Geometry check sheet. Reference: the model listing, model coordinates, mm. Round coordinates to 2 decimals unless told otherwise and drop trailing zeros. Write each loop counter-clockwise with the first axis right and the second up, starting at its lowest first coordinate (ties: lowest second). Pieces come first, ordered by that corner, then holes. Notation, with made-up numbers: (70.5, 16.5) - (98.5, 16.5) arc R13 cw to (98.5, 28.5) - close; hole circle Ø3 at (-22.5, 31). An arc over 180 degrees is marked (long way). Return JSON: item names as keys, results as strings.
```python
from build123d import *

# Parameters (mm, degrees)
SKETCH014_W            = 103
SKETCH014_H            = 207
PAD006_DEPTH           = 18
POCKET008_DEPTH        = 16
LINEARPATTERN_COUNT    = 4
LINEARPATTERN_PITCH    = 18
POCKET009_DEPTH        = 16
LINEARPATTERN001_COUNT = 2
LINEARPATTERN001_PITCH = 24
POCKET010_DEPTH        = 11.5
SKETCH019_W            = 55
SKETCH019_H            = 79
POCKET011_DEPTH        = 15
POCKET012_DEPTH        = 100
POCKET012_DEPTH_BACK   = 100
POCKET013_DEPTH        = 16
FILLET003_R            = 1
FILLET004_R            = 5
FILLET005_R            = 1
FILLET006_R            = 0.75


with BuildPart() as part:
    # Sketch014 → Pad006 (new body)
    with BuildSketch(Plane.XY):
        Rectangle(SKETCH014_W, SKETCH014_H)
    extrude(amount=PAD006_DEPTH)

    # Sketch015 (on Face6 of Pad006) → Pocket008 (cut)
    with BuildSketch(Plane(origin=(0, 90, 18), x_dir=(1, 0, 0), z_dir=(0, 0, 1))):
        with BuildLine():
            ThreePointArc((-40, 8), (-48, 0), (-40, -8))
            Line((-40, -8), (40, -8))
            ThreePointArc((40, -8), (48, 0), (40, 8))
            Line((-40, 8), (40, 8))
        make_face()
    pocket008 = extrude(amount=-POCKET008_DEPTH, mode=Mode.SUBTRACT)

    # LinearPattern: Pocket008 ×4
    with Locations(*[(0, -i * LINEARPATTERN_PITCH, 0) for i in range(1, LINEARPATTERN_COUNT)]):
        add(pocket008, mode=Mode.SUBTRACT)

    # Sketch017 → Pocket009 (cut)
    with BuildSketch(Plane(origin=(-15, 15, 18), x_dir=(1, 0, 0), z_dir=(0, 0, 1))):
        with BuildLine():
            Line((-23.5, 11), (23.5, 11))
            Line((23.5, 11), (15.797717, 0))
            Line((15.797717, 0), (23.5, -11))
            Line((23.5, -11), (-23.5, -11))
            ThreePointArc((-23.5, 11), (-34.5, 0), (-23.5, -11))
        make_face()
    pocket009 = extrude(amount=-POCKET009_DEPTH, mode=Mode.SUBTRACT)

    # LinearPattern001: Pocket009 ×2
    with Locations(*[(0, -i * LINEARPATTERN001_PITCH, 0) for i in range(1, LINEARPATTERN001_COUNT)]):
        add(pocket009, mode=Mode.SUBTRACT)

    # Sketch018 (on Face5 of LinearPattern001) → Pocket010 (cut)
    with BuildSketch(Plane.XY.offset(18)):
        with BuildLine():
            Line((48.255785, 16.86923), (48.255785, -41.13077))
            Line((48.255785, -41.13077), (43.255785, -41.13077))
            ThreePointArc((24.255785, -41.13077), (33.755784, -50.63077), (43.255785, -41.13077))
            Line((24.255785, -41.13077), (19.255785, -41.13077))
            Line((19.255785, -41.13077), (19.255785, 16.86923))
            Line((24.255785, 16.86923), (19.255785, 16.86923))
            ThreePointArc((43.255785, 16.86923), (33.755785, 26.36923), (24.255785, 16.86923))
            Line((43.255785, 16.86923), (48.255785, 16.86923))
        make_face()
    extrude(amount=-POCKET010_DEPTH, mode=Mode.SUBTRACT)

    # Sketch019 (on Face5 of Pocket010) → Pocket011 (cut)
    with BuildSketch(Plane.XY.offset(18)):
        with Locations((-22, -62)):
            Rectangle(SKETCH019_W, SKETCH019_H)
    extrude(amount=-POCKET011_DEPTH, mode=Mode.SUBTRACT)

    # Sketch020 (on Face46 of Pocket011) → Pocket012 (cut, two sides)
    with BuildSketch(Plane.XY.offset(3)) as pocket012_sk:
        with BuildLine():
            ThreePointArc((-35.75, -103.5), (-22, -117.25), (-8.25, -103.5))
            Line((-8.25, -103.5), (-8.25, -77.166667))
            ThreePointArc((-8.25, -77.166667), (-22, -63.416667), (-35.75, -77.166667))
            Line((-35.75, -103.5), (-35.75, -77.166667))
        make_face()
    extrude(amount=-POCKET012_DEPTH, mode=Mode.SUBTRACT)
    extrude(pocket012_sk.sketch, amount=POCKET012_DEPTH_BACK, mode=Mode.SUBTRACT)

    # Sketch021 (on Face5 of Pocket012) → Pocket013 (cut)
    with BuildSketch(Plane.XY.offset(18)):
        with BuildLine():
            ThreePointArc((7.5, -80.504131), (28.5, -101.504131), (49.5, -80.504131))
            Line((49.5, -80.504131), (49.5, -73.202981))
            ThreePointArc((49.5, -73.202981), (28.5, -52.202981), (7.5, -73.202981))
            Line((7.5, -80.504131), (7.5, -73.202981))
        make_face()
    extrude(amount=-POCKET013_DEPTH, mode=Mode.SUBTRACT)

    # Fillet003
    fillet003_edges = [part.edges().sort_by_distance(p)[0] for p in [
        (-42.625, -101.5, 18),
        (-49.5, -62, 18),
        (-22, -22.5, 18),
        (5.5, -62, 18),
        (-1.375, -101.5, 18),
    ]]
    fillet(fillet003_edges, radius=FILLET003_R)

    # Fillet004
    fillet004_edges = [part.edges().sort_by_distance(p)[0] for p in [
        (28.5, -52.202981, 2),
    ]]
    fillet(fillet004_edges, radius=FILLET004_R)

    # Fillet005
    fillet005_edges = [part.edges().sort_by_distance(p)[0] for p in [
        (48.255785, -12.13077, 18),
        (19.255785, -12.13077, 18),
    ]]
    fillet(fillet005_edges, radius=FILLET005_R)

    # Fillet006
    fillet006_edges = [part.edges().sort_by_distance(p)[0] for p in [
        (0, 80, 18),
        (-48, 72, 18),
        (0, 64, 18),
        (48, 72, 18),
        (0, 62, 18),
        (-48, 54, 18),
        (0, 46, 18),
        (48, 54, 18),
        (0, 44, 18),
        (-48, 36, 18),
        (0, 28, 18),
        (48, 36, 18),
        (0, 98, 18),
        (-48, 90, 18),
        (0, 82, 18),
        (48, 90, 18),
    ]]
    fillet(fillet006_edges, radius=FILLET006_R)


solid = part.part
```
(1) Material ranges on line 1 along X through (y, z) = (-60.5, 8.75); line 2 along Y through (x, z) = (15, 6); line 3 along Y through (x, z) = (18.5, 5.75), recorded low to high. Write a range as [from, to].
Response values:
{"line 1": "x = [-51.5, -49.5], [5.5, 11.78], [45.22, 51.5]", "line 2": "y = [-103.5, -96.46], [-57.25, 28], [44, 46], [62, 64], [80, 82], [98, 103.5]", "line 3": "y = [-103.5, -98.79], [-54.92, 28], [44, 46], [62, 64], [80, 82], [98, 103.5]"}
(2) Section check C-C, the plane y = 10. Enter the section's corners in (x, z).
Response values:
{"outline": "(-51.5, 0) - (51.5, 0) - (51.5, 18) - (49.26, 18) arc R1 ccw to (48.26, 17) - (48.26, 6.5) - (19.26, 6.5) - (19.26, 17) arc R1 ccw to (18.26, 18) - (4.3, 18) - (4.3, 2) - (-48.3, 2) - (-48.3, 18) - (-51.5, 18) - close"}
(3) Release check for a two-part mould opening along Y. For faces 1 (the face through (-21.7, -63.42, 1.52)), 2 (the face through (11, 8, 18)), 3 (the face through (5, 21, 10)) record: pulls with the +Y half, pulls with the -Y half, needs draft (parallel to the pull), parting line crosses it, or undercut.
Response values:
{"face 1": "pulls with the -Y half", "face 2": "needs draft", "face 3": "undercut"}
(4) Section check A-A, the plane y = 54. Enter the section's corners in (x, z), plus the area to 3 significant figures.
Response values:
{"outline": "(-51.5, 0) - (51.5, 0) - (51.5, 18) - (48.75, 18) arc R0.75 ccw to (48, 17.25) - (48, 2) - (-48, 2) - (-48, 17.25) arc R0.75 ccw to (-48.75, 18) - (-51.5, 18) - close", "area": "318 mm^2"}
(5) Section check B-B, the plane z = 10.75. Give the number of separate pieces and of enclosed holes in the cut face, plus the area to 3 significant figures.
Response values:
{"separate pieces": "1", "enclosed holes": "8", "area": "5,060 mm^2"}
(6) Gauge pin test, flat ends, axial feed: pin 1 (3 mm diameter, centred on x = 18.5, y = -79.5, fed in from +Z); pin 2 (17.5 mm diameter, centred on x = 3.5, y = 87.5, fed in from +Z); pin 3 (4 mm diameter, centred on x = -35, y = -56.5, fed in from +Z); pin 4 (4 mm diameter, centred on x = -14, z = 12.5, fed in from -Y). Record the tip position at first contact, or that the pin passes through.
Response values:
{"pin 1": "stops at z = 2", "pin 2": "stops at z = 18", "pin 3": "stops at z = 3", "pin 4": "stops at y = -22.5"}
